from build123d import *
from build123d.topology import SkipClean

# Parameters (mm, degrees)
SKETCH1_R           = 240
BOSS_EXTRUDE1_DEPTH = 10
BOSS_EXTRUDE2_START = 102.52
SKETCH2_R           = 240
SKETCH2_R_2         = 230
BOSS_EXTRUDE2_DEPTH = 102.52
CUT_EXTRUDE1_START  = -112.52
CUT_EXTRUDE1_DEPTH  = 112.52
BOSS_EXTRUDE4_START = 6
BOSS_EXTRUDE4_DEPTH = 6
CUT_EXTRUDE2_DEPTH  = 348.598906788
BOSS_EXTRUDE6_START = 10
BOSS_EXTRUDE6_DEPTH = 10
CUT_EXTRUDE3_START  = -118.52
CUT_EXTRUDE3_DEPTH  = 118.52


# Read off the part's stored shape, not the designer's step: Cut-Extrude1
with BuildPart() as part:
    # Sketch1 → Boss-Extrude1 (new body)
    with BuildSketch(Plane.XY.offset(65)):
        Circle(SKETCH1_R)
    extrude(amount=BOSS_EXTRUDE1_DEPTH)

    # Sketch2 → Boss-Extrude2 (add)
    with BuildSketch(Plane(origin=(0, 0, 65), x_dir=(-1, 0, 0), z_dir=(0, 0, -1)).offset(BOSS_EXTRUDE2_START)):
        Circle(SKETCH2_R)
        Circle(SKETCH2_R_2, mode=Mode.SUBTRACT)
    extrude(amount=-BOSS_EXTRUDE2_DEPTH)

    # Cut-Extrude1 outline → Cut-Extrude1 (cut)
    with BuildSketch(Plane(origin=(0, 0, -37.52), x_dir=(-1, 0, 0), z_dir=(0, 0, -1)).offset(CUT_EXTRUDE1_START)):
        with BuildLine():
            ThreePointArc((-87.384683401, -223.526099386), (232.916203487, -57.879548662), (27.411033925, 238.429518347))
            Line((27.411033925, 238.429518347), (27.411033925, -223.526099386))
            Line((27.411033925, -223.526099386), (-87.384683401, -223.526099386))
        make_face()
    extrude(amount=CUT_EXTRUDE1_DEPTH, mode=Mode.SUBTRACT)

    # Sketch5 → Boss-Extrude4 (add)
    with SkipClean():  # the faces are left unmerged after this step: merging them gives an invalid solid
        with BuildSketch(Plane(origin=(0, 0, -37.52), x_dir=(-1, 0, 0), z_dir=(0, 0, -1)).offset(BOSS_EXTRUDE4_START)):
            with BuildLine():
                Line((27.411033925, 228.360756741), (27.411033925, 238.429518347))
                ThreePointArc((27.411033925, 238.429518347), (-173.515297538, 165.808448277), (-236.939158864, -38.207787126))
                Line((-236.939158864, -38.207787126), (-226.804243794, -38.207787126))
                ThreePointArc((-226.804243794, -38.207787126), (-166.445517153, 158.732132285), (27.411033925, 228.360756741))
            make_face()
        extrude(amount=-BOSS_EXTRUDE4_DEPTH)

    # Sketch7 → Cut-Extrude2 (cut, through all)
    with SkipClean():  # the faces are left unmerged after this step: merging them gives an invalid solid
        with BuildSketch(Plane(origin=(0, 0, 0), x_dir=(0, 0, -1), z_dir=(1, 0, 0))):
            Polygon((-26.398, -50.207787126), (37.52, -50.207787126), (43.52, -50.207787126), (43.52, -37.967787126), (-27.418, -37.967787126), (-27.418, -49.187787126), (-27.418, -50.207787126), align=None)
        extrude(amount=CUT_EXTRUDE2_DEPTH, mode=Mode.SUBTRACT)

    # Sketch9 → Boss-Extrude6 (add)
    with SkipClean():  # the faces are left unmerged after this step: merging them gives an invalid solid
        with BuildSketch(Plane(origin=(0, 0, -43.52), x_dir=(-1, 0, 0), z_dir=(0, 0, -1)).offset(BOSS_EXTRUDE6_START)):
            with BuildLine():
                Line((-226.844543996, -37.967787126), (-236.977735538, -37.967787126))
                ThreePointArc((-236.977735538, -37.967787126), (-173.431306933, 165.896298258), (27.411033925, 238.429518347))
                Line((27.411033925, 238.429518347), (27.411033925, -37.967787126))
                Line((27.411033925, -37.967787126), (-226.844543996, -37.967787126))
            make_face()
        extrude(amount=-BOSS_EXTRUDE6_DEPTH)

    # Sketch10 → Cut-Extrude3 (cut)
    with BuildSketch(Plane.XY.offset(75).offset(CUT_EXTRUDE3_START)):
        with BuildLine():
            Line((-27.411033925, 238.429518347), (-27.411033925, -223.526099386))
            Line((-27.411033925, -223.526099386), (87.384683401, -223.526099386))
            ThreePointArc((87.384683401, -223.526099386), (232.916203487, 57.879548662), (-27.411033925, 238.429518347))
        make_face()
    extrude(amount=CUT_EXTRUDE3_DEPTH, mode=Mode.SUBTRACT)


solid = part.part
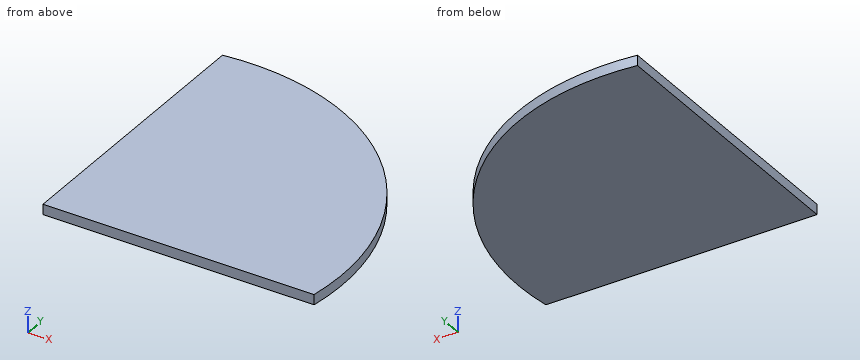
Can you work these out from the model? Positions are in its coordinate system, mm. Coordinates: 2 decimals unless noted, no trailing zeros. Loops run counter-clockwise (first coordinate to the right, second up) from the corner with the lowest first, then second, coordinate; pieces in that order, holes last. Notation, with made-up numbers: (52.5, 73) - (104.5, 73) arc R10 ccw to (104.5, 87) - close; hole circle Ø5 at (82, 11.5). An arc over 180 degrees is marked (long way). Answer as a JSON object with one key per item and string values. Group by question number.
Item 1: For pin 1 (4 mm diameter, centred on x = 61.5, z = -48, fed in from +Y); pin 2 (1.5 mm diameter, centred on x = 134.5, z = -49, fed in from +Y), each with a flat end and sliding along its axis, tell me the tip position at first contact or that it passes through.
Item 2: If we section it at A-A (z = -51): List the corners of the cut face in (x, y) for me, plus the area to 3 significant figures.
Item 3: If we section it at B-B (x = 217): List the corners of the cut face in (y, z) for me, plus the area to 3 significant figures.
Item 4: If I drill on L1, parallel to X at y = -2, z = -50.75; L2, parallel to Y at x = 1, z = -47.5; L3, parallel to Y at x = 185.5, z = -49.25, over which ranges is the centre line in solid material (lowest first)? Write a range as from..to.
Item 5: If we section it at C-C (y = 83.5): List the corners of the cut face in (x, z) for me.
Returned:
{
 "1": {"pin 1": "stops at y = 232.51", "pin 2": "stops at y = 199.28"},
 "2": {"outline": "(-27.41, -37.97) - (236.98, -37.97) arc R240 ccw to (-27.41, 238.43) - close", "area": "61,900 mm²"},
 "3": {"outline": "(-37.97, -53.52) - (102.52, -53.52) - (102.52, -43.52) - (-37.97, -43.52) - close", "area": "1,400 mm²"},
 "4": {"L1": "x = -27.41..239.99", "L2": "y = -37.97..240", "L3": "y = -37.97..152.28"},
 "5": {"outline": "(-27.41, -53.52) - (225.01, -53.52) - (225.01, -43.52) - (-27.41, -43.52) - close"}
}
